Could you check a few things on this drawing? It's one solid part, dimensions in mm from its lowest x, y, z. A direction names the side the tool comes from. Give positions to 0.01 mm unless a question says otherwise; leave off trailing zeros. Write each loop counter-clockwise with the first axis right and the second up, starting at its lowest first coordinate (ties: lowest second). Pieces come first, ordered by that corner, then holes.
1. I'm going to push flat-ended pins straight in: pin 1 (6 mm diameter, centred on x = 6.5, y = 20.5, fed in from +Z); pin 2 (8 mm diameter, centred on y = 4.5, z = 15, fed in from -X). Where does each tip first touch, or does it pass through?
2. Thinking about a two-plate mould opening in Y: for the marked faces 3, 4, 5 and 6, which applies, pulls with the +Y half, pulls with the -Y half, needs draft (parallel to the pull), parting line crosses it, or undercut?
3. On a 3-axis mill with a long thin cutter (end or side, diameter ignored), from which of +Z, -Z, +X, -X, +Y, -Y can I reach the whole of each face in a straight line? I mean the marked faces 1 and 2. Say none if no direction works.
4. If I drill on probe 1 along Y at (x, z) = (11.43, 1.25) (3 decimals); probe 2 along Z at (x, y) = (17.5, 21.75); probe 3 along X at (y, z) = (9, 2.75), over which ranges is the centre line in solid material (lowest first)?
5. Suppose I cut it at C-C (y = 12.7). Please give me the cut outline in (x, z) (3 decimals).
6. Suppose I cut it at A-A (x = 11.43). Please give me the cut outline in (y, z) (3 decimals), and give its area (3 significant figures).
7. Suppose I cut it at B-B (z = 12.7). Please give me the cut outline in (x, y) (3 decimals), and give its area (3 significant figures).
8. Suppose I cut it at D-D (x = 23.75). Please give me the cut outline in (y, z) (3 decimals).
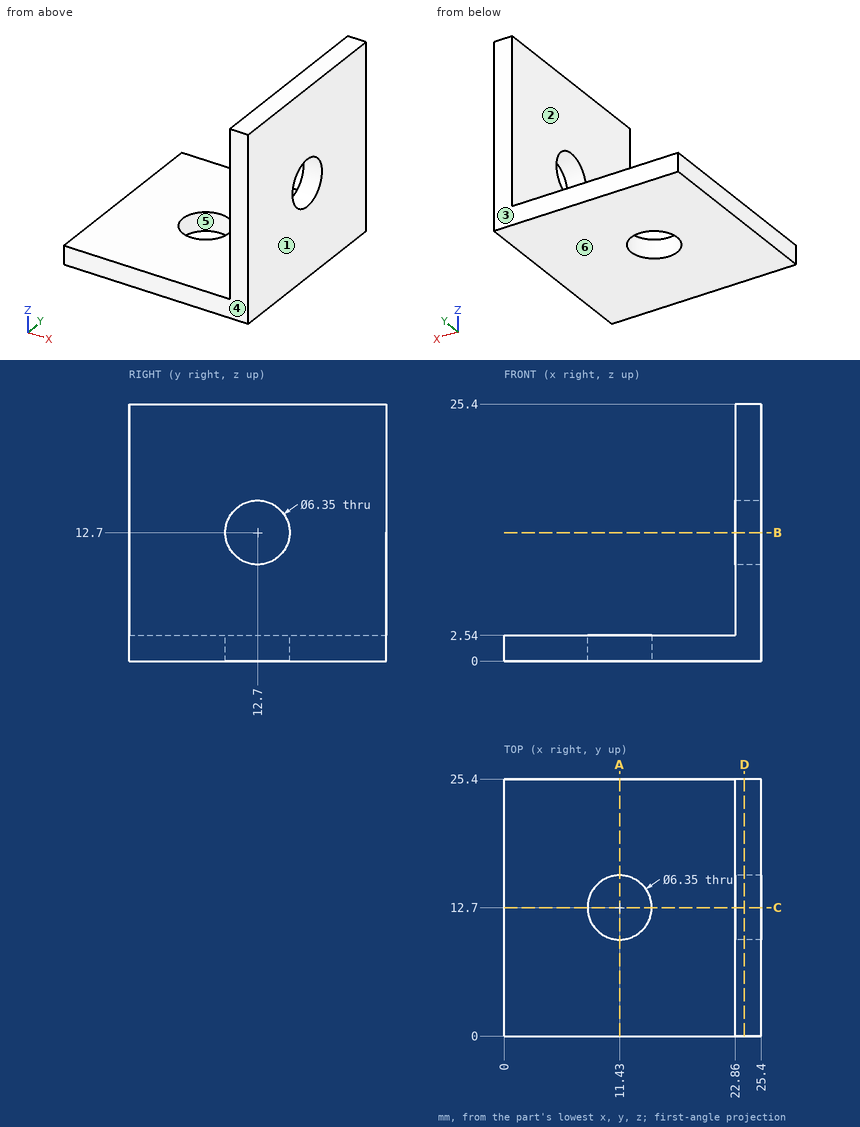
Checks:
1. pin 1: stops at z = 2.54
1. pin 2: stops at x = 22.86
2. face 3: pulls with the +Y half
2. face 4: pulls with the -Y half
2. face 5: undercut
2. face 6: needs draft
3. face 1: +Z, -Z, +X, +Y, -Y
3. face 2: +Z, -X, +Y, -Y
4. probe 1: y = 0 to 9.525, 15.875 to 25.4
4. probe 2: z = 0 to 2.54
4. probe 3: x = 22.86 to 25.4
5. outline: (0, 0) - (8.255, 0) - (8.255, 2.54) - (0, 2.54) - close; (14.605, 0) - (25.4, 0) - (25.4, 9.525) - (22.86, 9.525) - (22.86, 2.54) - (14.605, 2.54) - close; (22.86, 15.875) - (25.4, 15.875) - (25.4, 25.4) - (22.86, 25.4) - close
6. outline: (0, 0) - (9.525, 0) - (9.525, 2.54) - (0, 2.54) - close; (15.875, 0) - (25.4, 0) - (25.4, 2.54) - (15.875, 2.54) - close
6. area: 48.4 mm2
7. outline: (22.86, 0) - (25.4, 0) - (25.4, 9.525) - (22.86, 9.525) - close; (22.86, 15.875) - (25.4, 15.875) - (25.4, 25.4) - (22.86, 25.4) - close
7. area: 48.4 mm2
8. outline: (0, 0) - (25.4, 0) - (25.4, 25.4) - (0, 25.4) - close; hole circle Ø6.35 at (12.7, 12.7)
